Geometry check sheet. Reference: the model listing, model coordinates, mm. A direction names the side the tool comes from. Coordinates: 2 decimals unless noted, no trailing zeros. Write each loop counter-clockwise with the first axis right and the second up, starting at its lowest first coordinate (ties: lowest second). Pieces come first, ordered by that corner, then holes. Notation, with made-up numbers: (67.5, 16) -> (71.5, 16) arc R18 cw to (71.5, 28) -> close; hole circle Ø9 at (40.5, 9.25). An arc over 180 degrees is marked (long way). Answer in a Markdown table with one row per item. Add a question column.
Q1. Section check B-B, the plane x = 65.54. Record the boundary of the cut face in (y, z), and give its area (3 significant figures).
Q2. Section check A-A, the plane y = -36.5. Record the boundary of the cut face in (x, z).
Q3. Section check D-D, the plane y = 0. Record the boundary of the cut face in (x, z) (3 decimals), and give its area (3 significant figures).
Q4. Gauge pin test, flat ends, axial feed: P1, Ø3.5, axis at y = 31, z = 34, coming from the -X side; P2, Ø5, axis at y = 2.5, z = 27, coming from the +X side (3 decimals); P3, Ø12, axis at x = -81.5, z = 21, coming from the -Y side; P4, Ø3, axis at x = -82.085, y = 0, coming from the -Z side. Record the tip position at first contact, or that the pin passes through.
Q5. Section check C-C, the plane z = 22. Record the boundary of the cut face in (x, y) (3 decimals).
Q6. Thickness scan on line 1 (Y direction, x = 0, z = 4); line 2 (Y direction, x = 65.54, z = 33.25); line 3 (X direction, y = -20, z = 33) (1 decimal). Record the ranges inside material, lowest first.
Q7. Tool access check on faces 1 (the face through (-39, -27.64, 33)), 2 (the face through (38, -27.64, 33)), 3 (the face through (79, 0, 0)), 4 (the face through (77.085, 0, 20)), 5 (the face through (27.52, 32, 34)). Record the directions out of +Z, -Z, +X, -X, +Y, -Y that give a thin tool (end or side, any length) a straight path to the whole face; none if there is none.
Q8. Release check for a two-part mould opening along X. For faces 6 (the face through (83.735, 0.52, 2.535)), 7 (the face through (72.085, 16, 33)), 8 (the face through (-72.085, 16, 33)), 9 (the face through (0, -31.5, 20)) record: pulls with the +X half, pulls with the -X half, needs draft (parallel to the pull), parting line crosses it, or undercut.
```python
from build123d import *

# Parameters (mm, degrees)
SKETCH2_W             = 5
SKETCH2_H             = 10
BOSS_EXTRUDE1_DEPTH   = 32
SKETCH2_W_2           = 10
SKETCH2_H_2           = 5
BOSS_EXTRUDE1_2_DEPTH = 32
BOSS_EXTRUDE1_3_DEPTH = 32
BOSS_EXTRUDE1_4_DEPTH = 32
SKETCH3_W             = 165
SKETCH3_H             = 55.28
BOSS_EXTRUDE2_DEPTH   = 3
SKETCH4_W             = 10
SKETCH4_H             = 3.86
BOSS_EXTRUDE3_DEPTH   = 3
SKETCH5_W             = 10
SKETCH5_H             = 5
BOSS_EXTRUDE4_DEPTH   = 10
SKETCH7_W             = 5
SKETCH7_H             = 10
BOSS_EXTRUDE5_DEPTH   = 10
SKETCH8_R             = 1.73
CUT_EXTRUDE1_DEPTH    = 6
SKETCH10_W            = 10
SKETCH10_H            = 8.5
SKETCH10_W_2          = 1.85
SKETCH10_H_2          = 10
BOSS_EXTRUDE6_DEPTH   = 3
SKETCH11_R            = 1.75
CUT_EXTRUDE3_DEPTH    = 36
SKETCH12_W            = 82.72
SKETCH12_H            = 54.46
SKETCH12_W_2          = 81.92
SKETCH12_H_2          = 53.66
CUT_EXTRUDE4_DEPTH    = 0.28
CUT_EXTRUDE5_DEPTH    = 4


with BuildPart() as part:
    # Sketch2 → Boss-Extrude1 (new body)
    with BuildSketch(Plane.XY):
        with Locations((-74.585, 0)):
            Rectangle(SKETCH2_W, SKETCH2_H)
    extrude(amount=BOSS_EXTRUDE1_DEPTH)



with BuildPart() as body_2:
    # Sketch2 → Boss-Extrude1 2 (new body)
    with BuildSketch(Plane.XY):
        with Locations((0, 29)):
            Rectangle(SKETCH2_W_2, SKETCH2_H_2)
    extrude(amount=BOSS_EXTRUDE1_2_DEPTH)


with BuildPart() as body_3:
    # Sketch2 → Boss-Extrude1 3 (new body)
    with BuildSketch(Plane.XY):
        with Locations((74.585, 0)):
            Rectangle(SKETCH2_W, SKETCH2_H)
    extrude(amount=BOSS_EXTRUDE1_3_DEPTH)


with BuildPart() as body_4:
    # Sketch2 → Boss-Extrude1 4 (new body)
    with BuildSketch(Plane.XY):
        with Locations((0, -29)):
            Rectangle(SKETCH2_W_2, SKETCH2_H_2)
    extrude(amount=BOSS_EXTRUDE1_4_DEPTH)


with BuildPart() as part_1:
    add(part.part)

    add(body_2.part)  # Boss-Extrude2 merges body 2

    add(body_3.part)  # Boss-Extrude2 merges body 3

    add(body_4.part)  # Boss-Extrude2 merges body 4
    # Sketch3 → Boss-Extrude2 (add)
    with BuildSketch(Plane.XY.offset(32)):
        Rectangle(SKETCH3_W, SKETCH3_H)
    extrude(amount=BOSS_EXTRUDE2_DEPTH)

    # Sketch4 → Boss-Extrude3 (add)
    with BuildSketch(Plane.XY.offset(32)):
        with Locations((0, 29.57)):
            Rectangle(SKETCH4_W, SKETCH4_H)
        with Locations((0, -29.57)):
            Rectangle(SKETCH4_W, SKETCH4_H)
    extrude(amount=BOSS_EXTRUDE3_DEPTH)

    # Sketch5 → Boss-Extrude4 (add)
    with BuildSketch(Plane(origin=(0, 5, 0), x_dir=(1, 0, 0), z_dir=(0, 1, 0))):
        with Locations((-82.085, -2.5)):
            Rectangle(SKETCH5_W, SKETCH5_H)
        with Locations((82.085, -2.5)):
            Rectangle(SKETCH5_W, SKETCH5_H)
    extrude(amount=-BOSS_EXTRUDE4_DEPTH)

    # Sketch7 → Boss-Extrude5 (add)
    with BuildSketch(Plane.ZY.offset(5)):
        with Locations((2.5, 36.5)):
            Rectangle(SKETCH7_W, SKETCH7_H)
        with Locations((2.5, -36.5)):
            Rectangle(SKETCH7_W, SKETCH7_H)
    extrude(amount=-BOSS_EXTRUDE5_DEPTH)

    # Sketch8 → Cut-Extrude1 (cut, through all)
    with BuildSketch(Plane.XY.offset(5)):
        with Locations((-82.085, 0)):
            Circle(SKETCH8_R)
        with Locations((0, -36.5)):
            Circle(SKETCH8_R)
        with Locations((82.085, 0)):
            Circle(SKETCH8_R)
        with Locations((0, 36.5)):
            Circle(SKETCH8_R)
    extrude(amount=-CUT_EXTRUDE1_DEPTH, mode=Mode.SUBTRACT)

    # Sketch10 → Boss-Extrude6 (add)
    with BuildSketch(Plane.XY.offset(35)):
        with Locations((32.52, 31.89)):
            Rectangle(SKETCH10_W, SKETCH10_H)
        with Locations((69.005, -20.32)):
            Rectangle(SKETCH10_W_2, SKETCH10_H_2)
    extrude(amount=-BOSS_EXTRUDE6_DEPTH)

    # Sketch11 → Cut-Extrude3 (cut, through all)
    with BuildSketch(Plane.XY.offset(35)):
        with Locations((32.52, 31.75)):
            Circle(SKETCH11_R)
        with Locations((65.54, -20.32)):
            Circle(SKETCH11_R)
    extrude(amount=-CUT_EXTRUDE3_DEPTH, mode=Mode.SUBTRACT)

    # Sketch12 → Cut-Extrude4 (cut)
    with BuildSketch(Plane.XY.offset(35)):
        with Locations((-30.625, 0)):
            Rectangle(SKETCH12_W, SKETCH12_H)
        with Locations((-30.625, 0)):
            Rectangle(SKETCH12_W_2, SKETCH12_H_2, mode=Mode.SUBTRACT)
    extrude(amount=-CUT_EXTRUDE4_DEPTH, mode=Mode.SUBTRACT)

    # Sketch13 → Cut-Extrude5 (cut, through all)
    with BuildSketch(Plane(origin=(0, 0, 32), x_dir=(-1, 0, 0), z_dir=(0, 0, -1))):
        Polygon((82.5, -27.64), (82.5, 27.64), (72.085, 27.64), (72.085, 5), (77.085, 5), (77.085, -5), (72.085, -5), (72.085, -27.64), align=None)
        Polygon((-82.5, 27.64), (-82.5, -27.64), (-72.085, -27.64), (-72.085, -5), (-77.085, -5), (-77.085, 5), (-72.085, 5), (-72.085, 27.64), align=None)
    extrude(amount=-CUT_EXTRUDE5_DEPTH, mode=Mode.SUBTRACT)


solid = part_1.part
```
Calculated:
| question | item | result |
|---|---|---|
| 1 | outline | (-27.64, 32) -> (-22.07, 32) -> (-22.07, 35) -> (-27.64, 35) -> close; (-18.57, 32) -> (27.64, 32) -> (27.64, 35) -> (-18.57, 35) -> close |
| 1 | area | 155 mm² |
| 2 | outline | (-5, 0) -> (-1.73, 0) -> (-1.73, 5) -> (-5, 5) -> close; (1.73, 0) -> (5, 0) -> (5, 5) -> (1.73, 5) -> close |
| 3 | outline | (-87.085, 0) -> (-83.815, 0) -> (-83.815, 5) -> (-87.085, 5) -> close; (-80.355, 0) -> (-72.085, 0) -> (-72.085, 32) -> (72.085, 32) -> (72.085, 0) -> (80.355, 0) -> (80.355, 5) -> (77.085, 5) -> (77.085, 35) -> (10.735, 35) -> (10.735, 34.72) -> (10.335, 34.72) -> (10.335, 35) -> (-71.585, 35) -> (-71.585, 34.72) -> (-71.985, 34.72) -> (-71.985, 35) -> (-77.085, 35) -> (-77.085, 5) -> (-80.355, 5) -> close; (83.815, 0) -> (87.085, 0) -> (87.085, 5) -> (83.815, 5) -> close |
| 3 | area | 848 mm² |
| 4 | P1 | stops at x = -5 |
| 4 | P2 | stops at x = 77.085 |
| 4 | P3 | stops at y = -5 |
| 4 | P4 | passes through |
| 5 | outline | (-77.085, -5) -> (-72.085, -5) -> (-72.085, 5) -> (-77.085, 5) -> close; (-5, -31.5) -> (5, -31.5) -> (5, -26.5) -> (-5, -26.5) -> close; (-5, 26.5) -> (5, 26.5) -> (5, 31.5) -> (-5, 31.5) -> close; (72.085, -5) -> (77.085, -5) -> (77.085, 5) -> (72.085, 5) -> close |
| 6 | line 1 | y = -41.5 to -38.23, -34.77 to -26.5, 26.5 to 34.77, 38.23 to 41.5 |
| 6 | line 2 | y = -27.64 to -22.07, -18.57 to 27.64 |
| 6 | line 3 | x = -72.1 to 63.8, 67.3 to 72.1 |
| 7 | face 1 | +Z, -Z, -X, -Y |
| 7 | face 2 | +Z, -Z, +X, -Y |
| 7 | face 3 | -Z, +X, -X, +Y, -Y |
| 7 | face 4 | +Z, +X, +Y, -Y |
| 7 | face 5 | +Z, -Z, +Y |
| 8 | face 6 | undercut |
| 8 | face 7 | pulls with the +X half |
| 8 | face 8 | pulls with the -X half |
| 8 | face 9 | needs draft |
